```python
from build123d import *
from build123d import SkipClean  # not in build123d's __all__

# Parameters (mm, degrees)
F0_W      = 63.5
F0_H      = 38.1
F0_R      = 2.0193
F1_DEPTH  = 63.5
F2_DEPTH  = 25.4
F3_R      = 2.0193
F4_DEPTH  = 25.4
F5_R      = 1.5875
F6_DEPTH  = 19.05
F7_R      = 1.5875
F8_DEPTH  = 20.32
F9_R      = 1.63195
F10_DEPTH = 63.501
F9_R_2    = 9.525
F11_DEPTH = 9.144
F12_DEPTH = 2.794
F13_R     = 9.525
F13_R_2   = 1.63195
F14_DEPTH = 9.144
F15_DEPTH = 2.794


with BuildPart() as f1:
    # F0 (on Top) → F1 (new body)
    with BuildSketch(Plane.XY):
        Rectangle(F0_W, F0_H)
        with Locations((-24.13, -11.43)):
            Circle(F0_R, mode=Mode.SUBTRACT)
        with Locations((24.13, -11.43)):
            Circle(F0_R, mode=Mode.SUBTRACT)
        with Locations((-24.13, 11.43)):
            Circle(F0_R, mode=Mode.SUBTRACT)
        with Locations((24.13, 11.43)):
            Circle(F0_R, mode=Mode.SUBTRACT)
        with Locations((-24.13, 11.43)):
            Circle(F0_R)
        with Locations((24.13, 11.43)):
            Circle(F0_R)
        with Locations((24.13, -11.43)):
            Circle(F0_R)
        with Locations((-24.13, -11.43)):
            Circle(F0_R)
    extrude(amount=F1_DEPTH)

    # F0 (on Top) → F2 (cut)
    with BuildSketch(Plane.XY):
        with Locations((24.13, 11.43)):
            Circle(F0_R)
        with Locations((24.13, -11.43)):
            Circle(F0_R)
        with Locations((-24.13, 11.43)):
            Circle(F0_R)
        with Locations((-24.13, -11.43)):
            Circle(F0_R)
    extrude(amount=F2_DEPTH, mode=Mode.SUBTRACT)

    # F3 (on face) → F4 (cut)
    with BuildSketch(Plane.XY.offset(63.5)):
        with Locations((-19.05, 11.43)):
            Circle(F3_R)
        with Locations((-19.05, -11.43)):
            Circle(F3_R)
        with Locations((19.05, 11.43)):
            Circle(F3_R)
        with Locations((19.05, -11.43)):
            Circle(F3_R)
    extrude(amount=-F4_DEPTH, mode=Mode.SUBTRACT)

    # F5 (on face) → F6 (cut)
    with BuildSketch(Plane.XY):
        with Locations((-4.445, 0)):
            Circle(F5_R)
        with Locations((4.445, 0)):
            Circle(F5_R)
    extrude(amount=F6_DEPTH, mode=Mode.SUBTRACT)

    # F7 (on face) → F8 (cut)
    with BuildSketch(Plane.XZ.offset(19.05)):
        with Locations((-4.445, 19.05)):
            Circle(F7_R)
        with Locations((4.445, 19.05)):
            Circle(F7_R)
    with SkipClean():  # cleaning this boolean's faces spoils the solid; the shape is the same uncleaned
        extrude(amount=-F8_DEPTH, mode=Mode.SUBTRACT)

    # F9 (on face) → F10 (cut, through all)
    with BuildSketch(Plane.YZ.offset(31.75)):
        with Locations((0, 27.1272)):
            Circle(F9_R)
    with SkipClean():  # cleaning this boolean's faces spoils the solid; the shape is the same uncleaned
        extrude(amount=-F10_DEPTH, mode=Mode.SUBTRACT)

    # F9 (on face) → F11 (cut)
    with BuildSketch(Plane.YZ.offset(31.75)):
        with Locations((0, 27.1272)):
            Circle(F9_R_2)
        with Locations((0, 27.1272)):
            Circle(F9_R, mode=Mode.SUBTRACT)
    with SkipClean():  # cleaning this boolean's faces spoils the solid; the shape is the same uncleaned
        extrude(amount=-F11_DEPTH, mode=Mode.SUBTRACT)

    # F9 (on face) → F12 (cut)
    with BuildSketch(Plane.YZ.offset(31.75)):
        with BuildLine():
            Line((19.05, 24.9238323502), (19.05, 29.3305676498))
            ThreePointArc((19.05, 29.3305676498), (0, 46.3042), (-19.05, 29.3305676498))
            Line((-19.05, 29.3305676498), (-19.05, 24.9238323502))
            ThreePointArc((-19.05, 24.9238323502), (0, 7.9502), (19.05, 24.9238323502))
        make_face()
        with Locations((0, 27.1272)):
            Circle(F9_R_2, mode=Mode.SUBTRACT)
    with SkipClean():  # cleaning this boolean's faces spoils the solid; the shape is the same uncleaned
        extrude(amount=-F12_DEPTH, mode=Mode.SUBTRACT)

    # F13 (on face) → F14 (cut)
    with BuildSketch(Plane(origin=(-31.75, 0, 0), x_dir=(0, -1, 0), z_dir=(-1, 0, 0))):
        with Locations((0, 27.1272)):
            Circle(F13_R)
        with Locations((0, 27.1272)):
            Circle(F13_R_2, mode=Mode.SUBTRACT)
    with SkipClean():  # cleaning this boolean's faces spoils the solid; the shape is the same uncleaned
        extrude(amount=-F14_DEPTH, mode=Mode.SUBTRACT)

    # F13 (on face) → F15 (cut)
    with BuildSketch(Plane(origin=(-31.75, 0, 0), x_dir=(0, -1, 0), z_dir=(-1, 0, 0))):
        with BuildLine():
            Line((19.05, 24.9238323502), (19.05, 29.3305676498))
            ThreePointArc((19.05, 29.3305676498), (0, 46.3042), (-19.05, 29.3305676498))
            Line((-19.05, 29.3305676498), (-19.05, 24.9238323502))
            ThreePointArc((-19.05, 24.9238323502), (0, 7.9502), (19.05, 24.9238323502))
        make_face()
        with Locations((0, 27.1272)):
            Circle(F13_R, mode=Mode.SUBTRACT)
    with SkipClean():  # cleaning this boolean's faces spoils the solid; the shape is the same uncleaned
        extrude(amount=-F15_DEPTH, mode=Mode.SUBTRACT)


solid = f1.part
```
Model file for the job. Use its own axes, mm. A direction names the side the tool comes from. Give positions to 0.01 mm unless a question says otherwise; leave off trailing zeros. Order: outer loops, then holes, each group sorted by start corner. A loop starts at its lowest first (then second) coordinate and runs counter-clockwise, first axis right, second up.
1) Wall check: probe 1 along X at (y, z) = (-11.5, 19.05); probe 2 along Y at (x, z) = (-19, 43). Give the ranges that are in metal, low to high.
2) Mould opens along X. For faces 1 (the cylindrical face through (-30.373, 0.391, 7.954)), 2 (the flat face through (31.75, 0, 7)), 3 (the cylindrical face through (-25.62, 12.79, 12.52)) say: +X half, -X half, draft (parallel to the pull), parting line (faces both ways), or undercut.
3) Saw through at A-A, the plane z = 51.5. Write the cut outline in (x, y), then the cut area to 3 significant figures.
4) Pin check, flat tips, straight feed: pin 1 (4 mm diameter, centred on y = 0, z = 27.13, fed in from -X); pin 2 (3.5 mm diameter, centred on x = 19.05, y = 11.43, fed in from +Z); pin 3 (1.2 mm diameter, centred on x = -23.5, y = -10.5, fed in from -Z). Stop position of each tip, or through.
5) Saw through at C-C, the plane y = -11.43. Count the separate pieces of the cut face and the enclosed holes in it, then the cut area to 3 significant figures.
6) 3-axis set-ups, long thin cutter, end or side, ignore diameter. For faces 4 (the cylindrical face through (-4.652, 1.574, 9.392)), 5 (the cylindrical face through (-17.124, -10.823, 50.978)), 6 (the flat face through (28.956, -9, 23)): which of +Z, -Z, +X, -X, +Y, -Y reach the whole face in a straight line?
7) Saw through at B-B, the plane x = 19.05. Write the cut outline in (y, z), then the cut area to 3 significant figures.
8) Saw through at D-D, the plane y = 11.43. Write the cut outline in (x, z).
Computed:
1. probe 1: x = -28.96 to -26.15, -22.11 to -6.03, -2.86 to 2.86, 6.03 to 22.11, 26.15 to 28.96
1. probe 2: y = -19.05 to -13.45, -9.41 to 9.41, 13.45 to 19.05
2. face 1: draft
2. face 2: +X half
2. face 3: undercut
3. outline: (-31.75, -19.05) - (31.75, -19.05) - (31.75, 19.05) - (-31.75, 19.05) - close; hole circle Ø4.04 at (-19.05, -11.43); hole circle Ø4.04 at (-19.05, 11.43); hole circle Ø4.04 at (19.05, -11.43); hole circle Ø4.04 at (19.05, 11.43)
3. area: 2,370 mm2
4. pin 1: stops at x = -22.61
4. pin 2: stops at z = 38.1
4. pin 3: stops at z = 25.4
5. separate pieces: 1
5. enclosed holes: 2
5. area: 3,430 mm2
6. face 4: -Z
6. face 5: +Z
6. face 6: +X
7. outline: (-19.05, 0) - (19.05, 0) - (19.05, 63.5) - (13.45, 63.5) - (13.45, 38.1) - (9.41, 38.1) - (9.41, 63.5) - (-9.41, 63.5) - (-9.41, 38.1) - (-13.45, 38.1) - (-13.45, 63.5) - (-19.05, 63.5) - close; hole circle Ø3.26 at (0, 27.13)
7. area: 2,210 mm2
8. outline: (-31.75, 0) - (-26.15, 0) - (-26.15, 25.4) - (-22.11, 25.4) - (-22.11, 0) - (22.11, 0) - (22.11, 25.4) - (26.15, 25.4) - (26.15, 0) - (31.75, 0) - (31.75, 11.73) - (28.96, 11.73) - (28.96, 42.53) - (31.75, 42.53) - (31.75, 63.5) - (21.07, 63.5) - (21.07, 38.1) - (17.03, 38.1) - (17.03, 63.5) - (-17.03, 63.5) - (-17.03, 38.1) - (-21.07, 38.1) - (-21.07, 63.5) - (-31.75, 63.5) - (-31.75, 42.53) - (-28.96, 42.53) - (-28.96, 11.73) - (-31.75, 11.73) - close
